from build123d import *

# Parameters (mm, degrees)
SKETCH1_W           = 1200
SKETCH1_H           = 2500
BOSS_EXTRUDE1_DEPTH = 1000
CUT_EXTRUDE1_DEPTH  = 1000
CUT_EXTRUDE4_DEPTH  = 2948.880594597
CUT_EXTRUDE6_DEPTH  = 600
SKETCH6_R           = 250
CUT_EXTRUDE7_DEPTH  = 120
SKETCH7_R           = 30
CUT_EXTRUDE9_DEPTH  = 2840.013913347
SKETCH8_R           = 250
CUT_EXTRUDE10_DEPTH = 2948.880594722


with BuildPart() as part:
    # Sketch1 → Boss-Extrude1 (new body)
    with BuildSketch(Plane(origin=(0, 0, 0), x_dir=(1, 0, 0), z_dir=(0, 1, 0))):
        with Locations((-600, 1250)):
            Rectangle(SKETCH1_W, SKETCH1_H)
    extrude(amount=BOSS_EXTRUDE1_DEPTH)

    # Sketch2 → Cut-Extrude1 (cut)
    with BuildSketch(Plane(origin=(0, 1000, 0), x_dir=(1, 0, 0), z_dir=(0, 1, 0))):
        with BuildLine():
            Line((-900, 1794.983443527), (-900, 2500))
            Line((-900, 2500), (-1200, 2500))
            Line((-1200, 2500), (-1200, 1040))
            ThreePointArc((-1200, 1040), (-1157.592226371, 1261.564683763), (-1036.363636364, 1451.809151015))
            ThreePointArc((-1036.363636364, 1451.809151015), (-935.339811358, 1610.346207058), (-900, 1794.983443527))
        make_face()
        with BuildLine():
            Line((0, 2500), (-300, 2500))
            Line((-300, 2500), (-300, 1794.983443527))
            ThreePointArc((-300, 1794.983443527), (-264.660188642, 1610.346207058), (-163.636363636, 1451.809151015))
            ThreePointArc((-163.636363636, 1451.809151015), (-42.407773629, 1261.564683763), (0, 1040))
            Line((0, 1040), (0, 2500))
        make_face()
        with BuildLine():
            Line((-600, 0), (-600, 440))
            ThreePointArc((-600, 440), (-755.291427062, 460.444504227), (-900, 520.384757729))
            Line((-900, 520.384757729), (-900, 0))
            Line((-900, 0), (-600, 0))
        make_face()
        with BuildLine():
            Line((-600, 440), (-600, 700))
            ThreePointArc((-600, 700), (-812.132034356, 787.867965644), (-900, 1000))
            Line((-900, 1000), (-900, 520.384757729))
            ThreePointArc((-900, 520.384757729), (-755.291427062, 460.444504227), (-600, 440))
        make_face()
        with BuildLine():
            ThreePointArc((-300, 1000), (-387.867965644, 1212.132034356), (-600, 1300))
            Line((-600, 1300), (-600, 700))
            ThreePointArc((-600, 700), (-387.867965644, 787.867965644), (-300, 1000))
        make_face()
        with BuildLine():
            Line((-600, 700), (-600, 1300))
            ThreePointArc((-600, 1300), (-812.132034356, 1212.132034356), (-900, 1000))
            ThreePointArc((-900, 1000), (-812.132034356, 787.867965644), (-600, 700))
        make_face()
        with BuildLine():
            ThreePointArc((-300, 1000), (-387.867965644, 787.867965644), (-600, 700))
            Line((-600, 700), (-600, 440))
            ThreePointArc((-600, 440), (-444.708572938, 460.444504227), (-300, 520.384757729))
            Line((-300, 520.384757729), (-300, 1000))
        make_face()
        with BuildLine():
            ThreePointArc((-300, 520.384757729), (-444.708572938, 460.444504227), (-600, 440))
            Line((-600, 440), (-600, 0))
            Line((-600, 0), (-300, 0))
            Line((-300, 0), (-300, 520.384757729))
        make_face()
    extrude(amount=-CUT_EXTRUDE1_DEPTH, mode=Mode.SUBTRACT)

    # Sketch3 → Cut-Extrude4 (cut, through all)
    with BuildSketch(Plane(origin=(0, 0, 0), x_dir=(0, 0, -1), z_dir=(1, 0, 0))):
        with BuildLine():
            Line((500, 1000), (0, 1000))
            Line((0, 1000), (0, 499.999997907))
            ThreePointArc((0, 499.999997907), (146.446608667, 853.553389853), (500, 1000))
        make_face()
        with BuildLine():
            Line((1040, 1000), (500, 1000))
            ThreePointArc((500, 1000), (682.574185835, 965.474668126), (839.93463424, 866.666666667))
            ThreePointArc((839.93463424, 866.666666667), (918.614858442, 817.262665937), (1009.901951359, 800))
            Line((1009.901951359, 800), (1040, 800))
            Line((1040, 800), (1040, 1000))
        make_face()
        Polygon((1451.809151015, 1000), (1040, 1000), (1040, 800), (2500, 800), (2500, 1000), (1794.983443527, 1000), align=None)
        Polygon((1040, 200), (1040, 0), (1451.809151015, 0), (1794.983443527, 0), (2500, 0), (2500, 200), align=None)
        with BuildLine():
            ThreePointArc((839.93463424, 133.333333333), (682.574185835, 34.525331874), (500, 0))
            Line((500, 0), (1040, 0))
            Line((1040, 0), (1040, 200))
            Line((1040, 200), (1009.901951359, 200))
            ThreePointArc((1009.901951359, 200), (918.614858442, 182.737334063), (839.93463424, 133.333333333))
        make_face()
        with BuildLine():
            ThreePointArc((500, 0), (146.446610147, 146.446608667), (0, 499.999997907))
            Line((0, 499.999997907), (0, 0))
            Line((0, 0), (500, 0))
        make_face()
    extrude(amount=-CUT_EXTRUDE4_DEPTH, mode=Mode.SUBTRACT)

    # Sketch5 → Cut-Extrude6 (cut)
    with BuildSketch(Plane(origin=(0, 0, -2500), x_dir=(-1, 0, 0), z_dir=(0, 0, -1))):
        Polygon((300, 800), (300, 626), (474, 800), align=None)
        Polygon((900, 800), (813, 713), (900, 626), align=None)
        Polygon((900, 374), (726, 200), (900, 200), align=None)
        Polygon((387, 287), (300, 200), (474, 200), align=None)
        Polygon((300, 374), (300, 200), (387, 287), align=None)
        Polygon((726, 800), (813, 713), (900, 800), align=None)
    extrude(amount=-CUT_EXTRUDE6_DEPTH, mode=Mode.SUBTRACT)

    # Sketch6 → Cut-Extrude7 (cut)
    with BuildSketch(Plane(origin=(0, 0, -2500), x_dir=(-1, 0, 0), z_dir=(0, 0, -1))):
        with Locations((600, 500)):
            Circle(SKETCH6_R)
    extrude(amount=-CUT_EXTRUDE7_DEPTH, mode=Mode.SUBTRACT)

    # Sketch7 → Cut-Extrude9 (cut, through all)
    with BuildSketch(Plane.ZY.offset(900)):
        with Locations((-2440, 500)):
            Circle(SKETCH7_R)
    extrude(amount=-CUT_EXTRUDE9_DEPTH, mode=Mode.SUBTRACT)

    # Sketch8 → Cut-Extrude10 (cut, through all)
    with BuildSketch(Plane(origin=(0, 0, 0), x_dir=(0, 0, -1), z_dir=(1, 0, 0))):
        with Locations((500, 500)):
            Circle(SKETCH8_R)
    extrude(amount=-CUT_EXTRUDE10_DEPTH, mode=Mode.SUBTRACT)


solid = part.part
Verification items for the finished model (mm, model axes). A direction names the side the tool comes from. Give positions to 0.01 mm unless a question says otherwise; leave off trailing zeros. Order: outer loops, then holes, each group sorted by start corner. A loop starts at its lowest first (then second) coordinate and runs counter-clockwise, first axis right, second up. Notation, with made-up numbers: M 89.5,28.5 L 102.5,28.5 A13 ccw 102.5,36.5 Z; hole C -10,36 d2. An arc over 180 degrees is marked long. Answer as a JSON object with one key per item and string values. Group by question number.
1) Mould release check, pull along Y, two halves, no side actions. Record for faces 1 (the face through (0, 715, -628)), 2 (the face through (-1047.817, 817.744, -917.398)), 3 (the face through (-838.455, 575.093, -2440.84)): released by +Y, released by -Y, zero draft, split by the parting line, or undercut.
2) Cross-section at C-C (z = -390). Enter the section's corners in (x, y).
3) Access from +Z, -Z, +X, -X, +Y, -Y to the whole of each face (thin tool, end or side, straight path). Record for faces 4 (the face through (-592, 200, -1600)), 5 (the face through (-900, 504, -2064)), 6 (the face through (-812, 714, -2204)), 7 (the face through (-388, 286, -2204)).
4) Cross-section at D-D (x = -220.5). Enter the section's corners in (y, z).
5) Cross-section at B-B (x = -600). Enter the section's corners in (y, z), then the cut area to 3 significant figures.
6) Scan lines: line 1 along Y through (x, z) = (-1028, -500); line 2 along Y through (x, z) = (-600, -2473); line 3 along X through (y, z) = (452.5, -196.5). Record each from-to range of solid material in increasing order. Write a range as [from, to].
7) Depth check by flat-ended pin: pin 1 Ø8 at (x, y) = (-823.5, 623) entering from +Z; pin 2 Ø12 at (x, y) = (-1041, 735) entering from +Z; pin 3 Ø1 at (y, z) = (739.5, -1936.5) entering from +X. Enter the tip coordinate at first touch or a pass-through.
8) Cross-section at A-A (z = -2440). Enter the section's corners in (x, y), then the cut area to 3 significant figures.
Result sheet:
{
 "1": {"face 1": "zero draft", "face 2": "released by +Y", "face 3": "undercut"},
 "2": {"outline": "M -1200,12.25 L -900,12.25 L -900,275.5 L -1200,275.5 Z; M -1200,724.5 L -900,724.5 L -900,987.75 L -1200,987.75 Z; M -300,12.25 L 0,12.25 L 0,275.5 L -300,275.5 Z; M -300,724.5 L 0,724.5 L 0,987.75 L -300,987.75 Z"},
 "3": {"face 4": "-Z, +X, -X, -Y", "face 5": "-Z, -X, +Y, -Y", "face 6": "-Z, -X, +Y", "face 7": "-Z, +X, -Y"},
 "4": {"outline": "M 133.33,-839.93 A250 cw 200,-1009.9 L 200,-1524.47 L 800,-1524.47 L 800,-1009.9 A250 cw 866.67,-839.93 A500 ccw long Z; hole C 500,-500 d500"},
 "5": {"outline": "M 200,-2500 L 250,-2500 L 250,-2380 L 750,-2380 L 750,-2500 L 800,-2500 L 800,-1300 L 200,-1300 Z", "area": "660,000 mm2"},
 "6": {"line 1": "y = [0, 250], [750, 1000]", "line 2": "y = [200, 250], [750, 800]", "line 3": "x = [-1200, -900], [-300, 0]"},
 "7": {"pin 1": "stops at z = -1195.56", "pin 2": "stops at z = -55.52", "pin 3": "stops at x = -413"},
 "8": {"outline": "M -900,374 L -726,200 L -474,200 L -300,374 L -300,470 L -351.81,470 A250 cw -848.19,470 L -900,470 Z; M -900,530 L -848.19,530 A250 cw -351.81,530 L -300,530 L -300,626 L -474,800 L -726,800 L -900,626 Z", "area": "97,000 mm2"}
}
